from build123d import *

# Parameters (mm, degrees)
PART2_EYEBROW_START                          = -6.52585
PART2_EYEBROW_WARNING_MODULE_MIRRORED_OU_W   = 14.224
PART2_EYEBROW_WARNING_MODULE_MIRRORED_OU_H   = 8.128
PART2_EYEBROW_WARNING_MODULE_MIRRORED_OU_W_2 = 18.2372
PART2_EYEBROW_WARNING_MODULE_MIRRORED_OU_H_2 = 18.2372
PART2_EYEBROW_WARNING_MODULE_MIRRORED_DEPTH  = 6.52585
SKETCH2_W                                    = 6.35
SKETCH2_H                                    = 6.35
CUT_EXTRUDE1_DEPTH                           = 3.175
FILLET1_R                                    = 3.175


# Read off the part's stored shape, not the designer's step: Part2^Eyebrow Warning Module_Mirrored
with BuildPart() as part:
    # Part2^Eyebrow Warning Module_Mirrored ou → Part2^Eyebrow Warning Module_Mirrored (new body)
    with BuildSketch(Plane.XY.offset(PART2_EYEBROW_START)):
        with BuildLine():
            Line((573.893747576, 540.0294), (560.050747576, 540.0294))
            ThreePointArc((560.050747576, 540.0294), (557.715880985, 540.996533409), (556.748747576, 543.3314))
            Line((556.748747576, 543.3314), (556.748747576, 549.021))
            Line((556.748747576, 549.021), (541.000747576, 549.021))
            Line((541.000747576, 549.021), (541.000747576, 494.411))
            Line((541.000747576, 494.411), (573.893747576, 494.411))
            Line((573.893747576, 494.411), (573.893747576, 499.5418))
            ThreePointArc((573.893747576, 499.5418), (574.860880985, 501.876666591), (577.195747576, 502.8438))
            Line((577.195747576, 502.8438), (620.829097092, 502.8438))
            Line((620.829097092, 502.8438), (620.829097092, 522.605))
            Line((620.829097092, 522.605), (577.195747576, 522.605))
            ThreePointArc((577.195747576, 522.605), (574.860880985, 523.572133409), (573.893747576, 525.907))
            Line((573.893747576, 525.907), (573.893747576, 540.0294))
        make_face()
        with Locations((548.874747576, 499.237)):
            Rectangle(PART2_EYEBROW_WARNING_MODULE_MIRRORED_OU_W, PART2_EYEBROW_WARNING_MODULE_MIRRORED_OU_H, mode=Mode.SUBTRACT)
        with Locations((566.019747576, 499.237)):
            Rectangle(PART2_EYEBROW_WARNING_MODULE_MIRRORED_OU_W, PART2_EYEBROW_WARNING_MODULE_MIRRORED_OU_H, mode=Mode.SUBTRACT)
        with Locations((548.874747576, 508.2286)):
            Rectangle(PART2_EYEBROW_WARNING_MODULE_MIRRORED_OU_W, PART2_EYEBROW_WARNING_MODULE_MIRRORED_OU_H, mode=Mode.SUBTRACT)
        with Locations((548.874747576, 517.2202)):
            Rectangle(PART2_EYEBROW_WARNING_MODULE_MIRRORED_OU_W, PART2_EYEBROW_WARNING_MODULE_MIRRORED_OU_H, mode=Mode.SUBTRACT)
        with Locations((566.019747576, 508.2286)):
            Rectangle(PART2_EYEBROW_WARNING_MODULE_MIRRORED_OU_W, PART2_EYEBROW_WARNING_MODULE_MIRRORED_OU_H, mode=Mode.SUBTRACT)
        with Locations((566.019747576, 517.2202)):
            Rectangle(PART2_EYEBROW_WARNING_MODULE_MIRRORED_OU_W, PART2_EYEBROW_WARNING_MODULE_MIRRORED_OU_H, mode=Mode.SUBTRACT)
        with Locations((586.974747576, 512.7244)):
            Rectangle(PART2_EYEBROW_WARNING_MODULE_MIRRORED_OU_W_2, PART2_EYEBROW_WARNING_MODULE_MIRRORED_OU_H_2, mode=Mode.SUBTRACT)
        with Locations((610.948497092, 512.7244)):
            Rectangle(PART2_EYEBROW_WARNING_MODULE_MIRRORED_OU_W_2, PART2_EYEBROW_WARNING_MODULE_MIRRORED_OU_H_2, mode=Mode.SUBTRACT)
        with Locations((548.874747576, 526.2118)):
            Rectangle(PART2_EYEBROW_WARNING_MODULE_MIRRORED_OU_W, PART2_EYEBROW_WARNING_MODULE_MIRRORED_OU_H, mode=Mode.SUBTRACT)
        with Locations((548.874747576, 535.2034)):
            Rectangle(PART2_EYEBROW_WARNING_MODULE_MIRRORED_OU_W, PART2_EYEBROW_WARNING_MODULE_MIRRORED_OU_H, mode=Mode.SUBTRACT)
        with Locations((566.019747576, 526.2118)):
            Rectangle(PART2_EYEBROW_WARNING_MODULE_MIRRORED_OU_W, PART2_EYEBROW_WARNING_MODULE_MIRRORED_OU_H, mode=Mode.SUBTRACT)
        with Locations((566.019747576, 535.2034)):
            Rectangle(PART2_EYEBROW_WARNING_MODULE_MIRRORED_OU_W, PART2_EYEBROW_WARNING_MODULE_MIRRORED_OU_H, mode=Mode.SUBTRACT)
        with Locations((548.874747576, 544.195)):
            Rectangle(PART2_EYEBROW_WARNING_MODULE_MIRRORED_OU_W, PART2_EYEBROW_WARNING_MODULE_MIRRORED_OU_H, mode=Mode.SUBTRACT)
    extrude(amount=PART2_EYEBROW_WARNING_MODULE_MIRRORED_DEPTH)

    # Sketch2 → Cut-Extrude1 (cut)
    with BuildSketch(Plane(origin=(0, 0, -6.52585), x_dir=(-1, 0, 0), z_dir=(0, 0, -1))):
        with Locations((-617.654097092, 519.43)):
            Rectangle(SKETCH2_W, SKETCH2_H)
    extrude(amount=-CUT_EXTRUDE1_DEPTH, mode=Mode.SUBTRACT)

    # Fillet1
    fillet1_edges = [part.edges().sort_by_distance(p)[0] for p in [
        (614.479097092, 522.224, -3.35085),
        (620.448097092, 516.255, -3.35085),
    ]]
    fillet(fillet1_edges, radius=FILLET1_R - 0.0001)  # a hair under: the kernel refuses the full size


solid = part.part
Check sheet for the modelled part. Datum: model origin and axes. Units: mm. A direction names the side the tool comes from. Give positions to 0.01 mm unless a question says otherwise; leave off trailing zeros. Write each loop counter-clockwise with the first axis right and the second up, starting at its lowest first coordinate (ties: lowest second). Pieces come first, ordered by that corner, then holes. Notation, with made-up numbers: (86.5, 81) -> (139.5, 81) arc R21 cw to (139.5, 107) -> close; hole circle Ø5 at (19, -33.75). An arc over 180 degrees is marked (long way). One line per item, written item: value. Start each with the question number.
Item 1: Section check C-C on x = 584. Record the cut outline in (y, z) (3 decimals), then the cut area to 3 significant figures.
Item 2: Section check A-A on y = 509. Record the cut outline in (x, z), then the cut area to 3 significant figures.
Item 3: Draft check along Y on faces 4 (the flat face through (566, 530.276, -3)), 5 (the cylindrical face through (620.443, 517.16, -4.306)), 6 (the flat face through (557, 494.411, -3)). Enter one of: +Y half, -Y half, draft (parallel to the pull), parting line (faces both ways), or undercut.
Item 4: Section check B-B on y = 532. Record the cut outline in (x, z), then the cut area to 3 significant figures.
Item 5: Material ranges on probe 1 along X at (y, z) = (535, -2.75); probe 2 along Y at (x, z) = (572, -2.75); probe 3 along X at (y, z) = (521.5, -2.25), recorded low to high. Write a range as from..to.
Item 6: Section check D-D on z = -2.5. State how many separate pieces and enclosed holes the cut face has, then the cut area to 3 significant figures.
Item 7: Gauge pin test, flat ends, axial feed: pin 1 (2 mm diameter, centred on x = 611, z = -5, fed in from +Y) (3 decimals); pin 2 (4 mm diameter, centred on x = 569, y = 511.5, fed in from -Z). Record the tip position at first contact, or that the pin passes through.
Item 8: Tool access check on faces 1 (the flat face through (549, 549.021, -3)), 2 (the flat face through (567, 540.029, -3)), 3 (the flat face through (549, 548.259, -3)). Record the directions out of +Z, -Z, +X, -X, +Y, -Y that give a thin tool (end or side, any length) a straight path to the whole face; none if there is none.
Results list:
1. outline: (502.844, -6.526) -> (503.606, -6.526) -> (503.606, 0) -> (502.844, 0) -> close; (521.843, -6.526) -> (522.605, -6.526) -> (522.605, 0) -> (521.843, 0) -> close
1. area: 9.95 mm²
2. outline: (541, -6.53) -> (541.76, -6.53) -> (541.76, 0) -> (541, 0) -> close; (555.99, -6.53) -> (558.91, -6.53) -> (558.91, 0) -> (555.99, 0) -> close; (573.13, -6.53) -> (577.86, -6.53) -> (577.86, 0) -> (573.13, 0) -> close; (596.09, -6.53) -> (601.83, -6.53) -> (601.83, 0) -> (596.09, 0) -> close; (620.07, -6.53) -> (620.83, -6.53) -> (620.83, 0) -> (620.07, 0) -> close
2. area: 97.3 mm²
3. face 4: undercut
3. face 5: +Y half
3. face 6: -Y half
4. outline: (541, -6.53) -> (541.76, -6.53) -> (541.76, 0) -> (541, 0) -> close; (555.99, -6.53) -> (558.91, -6.53) -> (558.91, 0) -> (555.99, 0) -> close; (573.13, -6.53) -> (573.89, -6.53) -> (573.89, 0) -> (573.13, 0) -> close
4. area: 29.0 mm²
5. probe 1: 541..541.76, 555.99..558.91, 573.13..573.89
5. probe 2: 494.41..495.17, 503.3..504.16, 512.29..513.16, 521.28..522.15, 530.28..531.14, 539.27..540.03
5. probe 3: 541..577.86, 596.09..601.83, 620.07..620.83
6. separate pieces: 1
6. enclosed holes: 13
6. area: 640 mm²
7. pin 1: y = 522.605
7. pin 2: z = -6.53
8. face 1: +Z, -Z, +X, -X, +Y
8. face 2: +Z, -Z, +X, +Y
8. face 3: +Z, -Z
